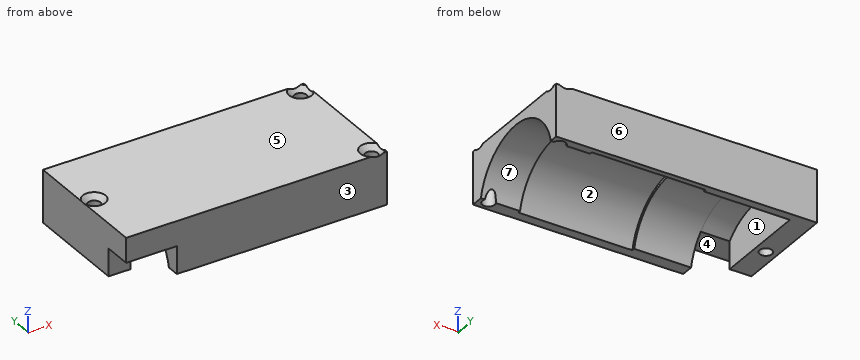
Autodesk Inventor part; units mm, degrees
ref_plane "Work Plane2" through (9.5, -31.75, -16.875) normal (1, 0, 0) x (0, 1, 0)
ref_plane "Work Plane3" through (-27.7, -29.75, -15.875) normal (-1, 0, 0) x (0, 0, 1)
ref_plane "Work Plane4" through (-41.5, -31.75, -7.5) normal (-1, 0, 0) x (0, 0, 1)
ref_plane "Work Plane1" through (0, -15.375, -1.5) normal (1, 0, 0) x (0, -1, 0)
sketch "Sketch1" plane through (0, -15.375, -1.5) normal (1, 0, 0) x (0, -1, 0)
  circle A0 centre (8, 0) radius 1.0564
  circle A1 centre (-8, 0) radius 1.0564
  circle A2 centre (0, 0) radius 5
  circle A3 centre (0, 0) radius 13.7
  line L0 (16.375, -1.5) -> (9.8735, -1.5)
  line L1 (16.375, -1.5) -> (16.375, 15.375)
  line L2 (16.375, 15.375) -> (-15.375, 15.375)
  line L3 (-15.375, 15.375) -> (-15.375, -1.5)
  line L4 (-15.375, -1.5) -> (-9.8735, -1.5)
  arc A4 (-6.7025, 2.019) -> (-9.8735, -1.5) centre (-8, 0) ccw
  arc A5 (6.7025, 2.019) -> (-6.7025, 2.019) centre (0, 0) ccw
  arc A6 (9.8735, -1.5) -> (6.7025, 2.019) centre (8, 0) ccw
  line L5 (16.375, -15.7) -> (-15.375, -15.7)
  line L6 (-15.375, -15.7) -> (-15.375, -3)
  line L7 (-15.375, -3) -> (16.375, -3)
  line L8 (16.375, -3) -> (16.375, -15.7)
  point P0 (0, -13.7)
  point P1 (13.3675, -3)
  point P2 (-13.3675, -3)
  dimension "d0" = 1.5
  dimension "d1" = 2
ref_plane "Work Plane2" through (9.5, -31.75, -16.875) normal (1, 0, 0) x (0, 1, 0)
extrude "Extrusion1" add sketch "Sketch1" along normal up to surface (9.5 mm away) contours A3 L7 L8 L5 L6
sketch "Sketch2" plane through (0, -15.375, -1.5) normal (-1, 0, 0) x (0, 0, 1)
  circle A0 centre (0, 0) radius 14.375
  line L0 (15.7, 15.375) -> (15.7, -16.375)
  line L1 (3, 15.375) -> (15.7, 15.375)
  line L2 (3, 13.3675) -> (3, 15.375)
  arc A1 (3, -13.3675) -> (3, 13.3675) centre (0, 0) ccw
  line L3 (3, -16.375) -> (3, -13.3675)
  line L4 (15.7, -16.375) -> (3, -16.375)
  point P0 (1.5, 15.375)
  point P1 (3, 14.0585)
  point P2 (3, -14.0585)
ref_plane "Work Plane3" through (-27.7, -29.75, -15.875) normal (-1, 0, 0) x (0, 0, 1)
extrude "Extrusion2" add sketch "Sketch2" along normal up to surface (27.7 mm away) contours A0 L2 L1 L0 L4 L3
sketch "Sketch3" plane through (-27.7, -15.375, -1.5) normal (-1, 0, 0) x (0, 0, 1)
  line L0 (-1.5, 11) -> (-1.5, 11.5)
  line L1 (-1.5, 11.5) -> (1.5, 11.5)
  line L2 (1.5, 11.5) -> (1.5, 11)
  line L3 (1.5, 11) -> (-1.5, 11)
  line L4 (1.5, -11.5) -> (1.5, -12)
  line L5 (1.5, -12) -> (-1.5, -12)
  line L6 (-1.5, -12) -> (-1.5, -11.5)
  line L7 (-1.5, -11.5) -> (1.5, -11.5)
  circle A0 centre (0, 0) radius 5
  circle A1 centre (0, 0) radius 13.7
  line L8 (15.7, -16.375) -> (3, -16.375)
  line L9 (15.7, 15.375) -> (15.7, -16.375)
  line L10 (3, 15.375) -> (15.7, 15.375)
  line L11 (3, 14.0585) -> (3, 15.375)
  arc A2 (3, -14.0585) -> (3, 14.0585) centre (0, 0) ccw
  line L12 (3, -16.375) -> (3, -14.0585)
  circle A3 centre (0, 0) radius 14.375
  circle A4 centre (0, 0) radius 13.7
  line L13 (15.7, 15.375) -> (3, 15.375)
  line L14 (15.7, 15.375) -> (3, 15.375)
  line L15 (3, 15.375) -> (3, -16.375)
  line L16 (3, -16.375) -> (15.7, -16.375)
  line L17 (15.7, -16.375) -> (15.7, 15.375)
  point P0 (1.5, 15.375)
  point P1 (3, -13.3675)
  point P2 (3, -14.0585)
  point P3 (3, 13.3675)
ref_plane "Work Plane4" through (-41.5, -31.75, -7.5) normal (-1, 0, 0) x (0, 0, 1)
extrude "Extrusion3" add sketch "Sketch3" along normal up to surface (13.8 mm away) contours L15 A2 A1 | L11 L10 L9 L8 L12 A2
sketch "Sketch4" plane through (-41.5, -15.375, -1.5) normal (-1, 0, 0) x (0, 0, 1)
  arc A0 (3, -13.3675) -> (3, 13.3675) centre (0, 0) ccw
  line L0 (3, -16.375) -> (3, -13.3675)
  line L1 (15.7, -16.375) -> (3, -16.375)
  line L2 (15.7, 15.375) -> (15.7, -16.375)
  line L3 (3, 15.375) -> (15.7, 15.375)
  line L4 (3, 13.3675) -> (3, 15.375)
  line L5 (15.7, 15.375) -> (3, 15.375)
  line L6 (3, -16.375) -> (15.7, -16.375)
  line L7 (15.7, 15.375) -> (9.7, 15.375)
  line L8 (9.7, 15.375) -> (9.7, -16.375)
  line L9 (9.7, -16.375) -> (15.7, -16.375)
  line L10 (15.7, -16.375) -> (15.7, 15.375)
  point P0 (1.5, 15.375)
  point P1 (9.7, -9.6747)
  point P2 (9.7, -16.375)
  dimension "d8" = 6
ref_plane "Work Plane5" through (-48.5, -20.375, -7.5) normal (1, 0, 0) x (0, 1, 0)
extrude "Extrusion4" add sketch "Sketch4" along normal up to surface (7 mm away) contours A0 L8 L3 L2 L1 | A0 L4 L3 L8
sketch "Sketch5" plane through (-48.5, -31.75, 14.2) normal (-1, 0, 0) x (0, 0, 1)
  line L0 (-12.7, 31.75) -> (-12.7, 29.7425)
  arc A0 (-6, 6.7003) -> (-12.7, 29.7425) centre (-15.7, 16.375) ccw
  line L1 (-6, 6.7003) -> (-6, 0)
  line L2 (-6, 0) -> (0, 0)
  line L3 (0, 0) -> (0, 31.75)
  line L4 (0, 31.75) -> (-12.7, 31.75)
  line L5 (-6, 0) -> (-6, 6.7003)
  arc A1 (-12.7, 3.0075) -> (-6, 6.7003) centre (-15.7, 16.375) ccw
  line L6 (-12.7, 0) -> (-12.7, 3.0075)
  line L7 (-6, 0) -> (-12.7, 0)
  line L8 (0, 0) -> (0, 31.75)
  line L9 (-12.7, 0) -> (0, 0)
  line L10 (0, 31.75) -> (-12.7, 31.75)
  line L11 (-12.7, 31.75) -> (-12.7, 0)
  line L12 (-12.7, 0) -> (0, 0)
  line L13 (0, 0) -> (0, 31.75)
  line L14 (-6, 6.7003) -> (-12.7, 6.7003)
  point P0 (-14.2, 31.75)
  point P1 (-6, 6.7003)
ref_plane "Work Plane6" through (-53.8, -31.75, -16.875) normal (-1, 0, 0) x (0, 0, 1)
extrude "Extrusion5" add sketch "Sketch5" along normal up to surface (5.3 mm away) contours L4 L3 L2 L1 A0 L0 | A0 L14 L11
sketch "Sketch6" plane through (9.5, -31.75, 14.2) normal (0, 0, 1) x (1, 0, 0)
  circle A0 centre (-2.3, 29.45) radius 1.55
  circle A1 centre (-2.3, 2.3) radius 1.55
  circle A2 centre (-60.65, 16.375) radius 1.55
  point P0 (-9.5, 31.75)
hole "Hole1" at (7.2, -2.3, 14.2) at (7.2, -29.45, 14.2) at (-51.15, -15.375, 14.2) direction (0, 0, -1) diameter 3 depth 14.5 countersink diameter 5.5 countersink angle 90
properties part number "right_motor_ceil"
Here's how the part is built. I have some questions about the finished solid (model axes, mm). Face numbers are marked on the shaded views. A direction names the side the tool comes from. Coordinates: 2 decimals unless noted, no trailing zeros. Order: outer loops, then holes, each group sorted by start corner. A loop starts at its lowest first (then second) coordinate and runs counter-clockwise, first axis right, second up. Notation, with made-up numbers: (-5.5, 61) - (4.5, 61) arc R25 cw to (4.5, 94) - close; hole circle Ø9 at (49.5, 46.25). An arc over 180 degrees is marked (long way). One line per question, with ' | ' between items. Start each with the question number.
1. Please list where these lines run through material, in increasing order: line 1 along X through (y, z) = (-29.45, 10); line 2 along Y through (x, z) = (7.2, 8); line 3 along Y through (x, z) = (7.2, 8.25). Write a range as [from, to].
2. If we section it at B-B (z = 6.5): Write out the boundary of the cut face in (x, y) (3 decimals).
3. If we section it at D-D (z = 9.75): Write out the boundary of the cut face in (x, y) (3 decimals), and give its area (3 significant figures).
4. I'm going to push flat-ended pins straight in: pin 1 Ø5.5 at (y, z) = (-10.5, 8) entering from +X; pin 2 Ø3.5 at (y, z) = (-29.5, 6) entering from -X; pin 3 Ø7.5 at (x, y) = (-45.5, -30) entering from -Z. Where does each tip first touch, or does it pass through?
5. Which directions (+Z, -Z, +X, -X, +Y, -Y) give clear straight access to the entire face, cutting with the end or side of a thin tool? Please do the marked faces 1, 2, 3 and 4.
6. If we section it at C-C (x = 7.2): Write out the boundary of the cut face in (y, z) (3 decimals).
7. If we mould it in two halves opening along Y, with no side actions, what happens to the marked faces 5, 6 and 7? For each: released by +Y, released by -Y, zero draft, split by the parting line, or undercut.
8. If we section it at A-A (x = -51.15): Write out the boundary of the cut face in (y, z) (3 decimals), and give its area (3 significant figures).
Model answer:
1) line 1: x = [-53.8, 5.7], [8.7, 9.5] | line 2: y = [-31.75, -30.95], [-27.95, -25.25], [-5.5, -3.8], [-0.8, 0] | line 3: y = [-31.75, -30.95], [-27.95, -25], [-5.75, -3.8], [-0.8, 0]
2) outline: (-53.8, -25.05) - (-48.5, -25.05) - (-48.5, -4.253) - (-27.7, -4.253) - (-27.7, -3.432) - (0, -3.432) - (0, -4.253) - (9.5, -4.253) - (9.5, 0) - (-53.8, 0) - close; (-41.5, -31.75) - (9.5, -31.75) - (9.5, -26.497) - (0, -26.497) - (0, -27.318) - (-27.7, -27.318) - (-27.7, -26.497) - (-41.5, -26.497) - close; hole circle Ø3 at (-51.15, -15.375); hole circle Ø3 at (7.2, -29.45); hole circle Ø3 at (7.2, -2.3)
3) outline: (-53.8, -31.75) - (9.5, -31.75) - (9.5, -23.193) - (0, -23.193) - (0, -24.324) - (-27.7, -24.324) - (-27.7, -23.193) - (-48.5, -23.193) - (-48.5, -7.557) - (-27.7, -7.557) - (-27.7, -6.426) - (0, -6.426) - (0, -7.557) - (9.5, -7.557) - (9.5, 0) - (-53.8, 0) - close; hole circle Ø3 at (-51.15, -15.375); hole circle Ø3 at (7.2, -29.45); hole circle Ø3 at (7.2, -2.3) | area: 1,020 mm²
4) pin 1: stops at x = -48.5 | pin 2: stops at x = -41.5 | pin 3: stops at z = 8.2
5) face 1: -Z, +X | face 2: -Z | face 3: +Z, -Z, +X, -X, -Y | face 4: -Z, -X, -Y
6) outline: (-31.75, 1.5) - (-30.95, 1.5) - (-30.95, 12.95) - (-31.75, 13.75) - close; (-27.95, 3.937) arc R13.7 cw to (-3.8, 5.829) - (-3.8, 12.95) - (-5.05, 14.2) - (-26.7, 14.2) - (-27.95, 12.95) - close; (-0.8, 1.5) - (0, 1.5) - (0, 13.75) - (-0.8, 12.95) - close
7) face 5: zero draft | face 6: released by +Y | face 7: undercut
8) outline: (-31.75, 8.2) - (-25.05, 8.2) - (-25.05, 1.5) - (-16.875, 1.5) - (-16.875, 12.95) - (-18.125, 14.2) - (-31.75, 14.2) - close; (-13.875, 1.5) - (0, 1.5) - (0, 14.2) - (-12.625, 14.2) - (-13.875, 12.95) - close | area: 319 mm²
